Design review of the part built by this model. Coordinates are the model's own, in mm. A direction names the side the tool comes from. Round coordinates to 2 decimals unless told otherwise and drop trailing zeros. Order: outer loops, then holes, each group sorted by start corner. A loop starts at its lowest first (then second) coordinate and runs counter-clockwise, first axis right, second up. Notation, with made-up numbers: (20, -23) - (61, -23) arc R22 ccw to (61, 2) - close; hole circle Ø3 at (9.5, 79). An arc over 180 degrees is marked (long way). Write item = value, one per line.
Autodesk Fusion 360 part; units mm, degrees
sketch "Sketch1" plane through (0, 0, 0) normal (0, 1, 0) x (1, 0, 0)
  circle A0 centre (0, 13.5) radius 9.75
  circle A1 centre (-11.6913, -6.75) radius 9.75
  circle A2 centre (11.6913, -6.75) radius 9.75
  line L0 (25.9808, -15) -> (0, 30)
  line L1 (0, 30) -> (-25.9808, -15)
  line L2 (-25.9808, -15) -> (25.9808, -15)
  circle A3 centre (0, 13.5) radius 12
  circle A4 centre (-11.6913, -6.75) radius 12
  circle A5 centre (11.6913, -6.75) radius 12
  circle A6 centre (0, 0) radius 2.5
  circle A7 centre (-11.6913, -6.75) radius 1.5
  circle A8 centre (11.6913, -6.75) radius 1.5
  circle A9 centre (0, 13.5) radius 1.5
  dimension "d1" = 19.5
  dimension "d2" = 13.5
  dimension "d4" = 360
  dimension "d5" = 30
  dimension "d6" = 24
  dimension "d8" = 360
  dimension "d9" = 5
  dimension "d14" = 3
  dimension "d16" = 360
extrude "Extrude1" add sketch "Sketch1" along normal blind 3 contours A0 L0 | A0 L0 A3 | A0 L0 L1 | A0 L0 L1 A3 | A0 L0 L1 A3 A4 A5 A6 | A0 L1 | A0 L1 A3 | L0 A3 A5 | L1 A3 A4 | A2 L0 A5 | A2 L0 L2 A3 A4 A5 A6 | A3 A5 | A1 L1 L2 A3 A4 A5 A6 | A1 L1 A4 | A3 A4 | A2 L0 L2 | A2 L0 | A3 A5 A6 | A1 L1 | A1 L1 L2 | A1 L1 L2 A4 | A3 A4 A6 | A2 L2 | A2 L2 A5 | A2 L0 L2 A5 | A1 L2 A4 | L2 A4 A5 | A4 A5 A6 | A1 L2 | A4 A5 | A7 | A8 | A9
extrude "Extrude2" add sketch "Sketch1" against normal blind 10 contours A0 L0 A3 | A0 L0 L1 A3 | A0 L0 L1 A3 A4 A5 A6 | A0 L1 A3 | L0 A3 A5 | L1 A3 A4 | A2 L0 A5 | A2 L0 L2 A3 A4 A5 A6 | A3 A5 | A1 L1 L2 A3 A4 A5 A6 | A1 L1 A4 | A3 A4 | A3 A5 A6 | A1 L1 L2 A4 | A3 A4 A6 | A2 L2 A5 | A2 L0 L2 A5 | A1 L2 A4 | L2 A4 A5 | A4 A5 A6 | A4 A5
extrude "Extrude3" cut sketch "Sketch1" along normal through all contours A7 | A8 | A9
Item 1: Take a section at A-A, the plane z = 6.75. State the section outline as (x, y) points.
Data:
outline = (-23.69, -10) - (-21.44, -10) - (-21.44, 0) - (-13.19, 0) - (-13.19, 3) - (-23.69, 3) - close; (-10.19, 0) - (-1.94, 0) - (-1.94, -10) - (1.94, -10) - (1.94, 0) - (10.19, 0) - (10.19, 3) - (-10.19, 3) - close; (13.19, 0) - (21.44, 0) - (21.44, -10) - (23.69, -10) - (23.69, 3) - (13.19, 3) - close
Item 2: Take a section at B-B, the plane z = -13.5. State the section outline as (x, y) points, and give its area (3 significant figures).
Data:
outline = (-12, -10) - (-9.75, -10) - (-9.75, 0) - (-1.5, 0) - (-1.5, 3) - (-12, 3) - close; (1.5, 0) - (9.75, 0) - (9.75, -10) - (12, -10) - (12, 3) - (1.5, 3) - close
area = 108 mm2
Item 3: Take a section at C-C, the plane x = 0. State the section outline as (y, z) points, and give its area (4 significant figures).
Data:
outline = (-10, -25.5) - (3, -25.5) - (3, -15) - (0, -15) - (0, -23.25) - (-10, -23.25) - close; (-10, -3.75) - (0, -3.75) - (0, -12) - (3, -12) - (3, -2.5) - (-10, -2.5) - close; (-10, 2.5) - (3, 2.5) - (3, 15) - (-10, 15) - close
area = 257.5 mm2
Item 4: Insertion check: P1, Ø6, axis at x = -2.5, y = -2, coming from the +Z side; P2, Ø4, axis at x = 11.69, z = 6.75, coming from the +Y side; P3, Ø2, axis at y = 1, z = -18, coming from the -X side; P4, Ø5, axis at x = 6, y = -1, coming from the +Z side. Each pin has a flat end and moves straight along its axis. Give the tip position at first contact, or say it passes through.
Data:
P1 = 17.03
P2 = 3
P3 = -11.48
P4 = 18.32
Item 5: Take a section at D-D, the plane y = 1. State the section outline as (x, z) points, and give its area (3 significant figures).
Data:
outline = (-14.48, -4.92) - (-11.5, -10.08) arc R12 ccw (long way) to (11.5, -10.08) - (14.48, -4.92) arc R12 ccw (long way) to (2.98, 15) - (-2.98, 15) arc R12 ccw (long way) to start; hole circle Ø3 at (-11.69, 6.75); hole circle Ø5 at (0, 0); hole circle Ø3 at (0, -13.5); hole circle Ø3 at (11.69, 6.75)
area = 1,360 mm2
Item 6: For line 1 along X through (y, z) = (0.9, 6.75); line 2 along X through (y, z) = (-2.75, 6.75); line 3 along X through (y, z) = (-6.25, 0), list the stretches that pass through material, from the lowest coordinate up. Write a range as [from, to].
Data:
line_1 = [-23.69, -13.19], [-10.19, 10.19], [13.19, 23.69]
line_2 = [-23.69, -21.44], [-1.94, 1.94], [21.44, 23.69]
line_3 = [-21.61, -18.73], [-4.66, -2.5], [2.5, 4.66], [18.73, 21.61]
Item 7: For faces 1 (the face through (-12.97, -3.409, -7.536)), 2 (the face through (13.08, 1.48, 6.18)), 3 (the face through (-12.961, -4.93, -2.917)), list the 3-axis set-ups (+Z, -Z, +X, -X, +Y, -Y) from which the entire face can be reached by the end or side of a thin tool; tool diameter is ignored.
Data:
face_1 = -X, +Y, -Y
face_2 = +Y, -Y
face_3 = -Y
Item 8: The part is to be moulded in two halves that separate along Z. For faces 4 (the face through (-22.236, -3.409, 12.477)), 5 (the face through (0, 1, -15)), 6 (the face through (0, -3, 15)), say which applies: +Z half, -Z half, draft (parallel to the pull), parting line (faces both ways), or undercut.
Data:
face_4 = parting line
face_5 = undercut
face_6 = +Z half
